```python
from build123d import *

# Parameters (mm, degrees)
SKETCH_1_R               = 40
EXTRUDE_1_DEPTH          = 5
SKETCH_2_R               = 31
EXTRUDE_2_DEPTH          = 12
SKETCH_3_R               = 26
CUT_EXTRUDE_1_DEPTH      = 15
SKETCH_4_R               = 31
EXTRUDE_3_DEPTH          = 3
SKETCH_6_R               = 2
CUT_EXTRUDE_3_DEPTH      = 5
PATTERN_CIRCULAR_1_COUNT = 4
SKETCH_7_R               = 20
CUT_EXTRUDE_4_DEPTH      = 10


with BuildPart() as part:
    # 草图1 → 凸台-拉伸1 (new body)
    with BuildSketch(Plane.XY):
        Circle(SKETCH_1_R)
    extrude(amount=EXTRUDE_1_DEPTH)

    # 草图2 → 凸台-拉伸2 (add)
    with BuildSketch(Plane.XY.offset(5)):
        Circle(SKETCH_2_R)
    extrude(amount=EXTRUDE_2_DEPTH)

    # 草图3 → 切除-拉伸1 (cut)
    with BuildSketch(Plane(origin=(0, 0, 0), x_dir=(-1, 0, 0), z_dir=(0, 0, -1))):
        Circle(SKETCH_3_R)
    extrude(amount=-CUT_EXTRUDE_1_DEPTH, mode=Mode.SUBTRACT)

    # 草图4 → 凸台-拉伸3 (add)
    with BuildSketch(Plane.XY.offset(17)):
        Circle(SKETCH_4_R)
    extrude(amount=EXTRUDE_3_DEPTH)

    # 草图6 → 切除-拉伸3 (cut)
    with BuildSketch(Plane(origin=(0, 0, 0), x_dir=(-1, 0, 0), z_dir=(0, 0, -1))):
        with Locations((0, 36)):
            Circle(SKETCH_6_R)
    cut_extrude_3 = extrude(amount=-CUT_EXTRUDE_3_DEPTH, mode=Mode.SUBTRACT)

    # 阵列(圆周)1: 切除-拉伸3 ×4 about axis
    pattern_circular_1_axis = Axis((0, 0, 0), (0, 0, 1))
    for i in range(1, PATTERN_CIRCULAR_1_COUNT):
        add(cut_extrude_3.rotate(pattern_circular_1_axis, i * 360 / PATTERN_CIRCULAR_1_COUNT), mode=Mode.SUBTRACT)

    # 草图7 → 切除-拉伸4 (cut)
    with BuildSketch(Plane.XY.offset(20)):
        Circle(SKETCH_7_R)
    extrude(amount=-CUT_EXTRUDE_4_DEPTH, mode=Mode.SUBTRACT)


solid = part.part
```
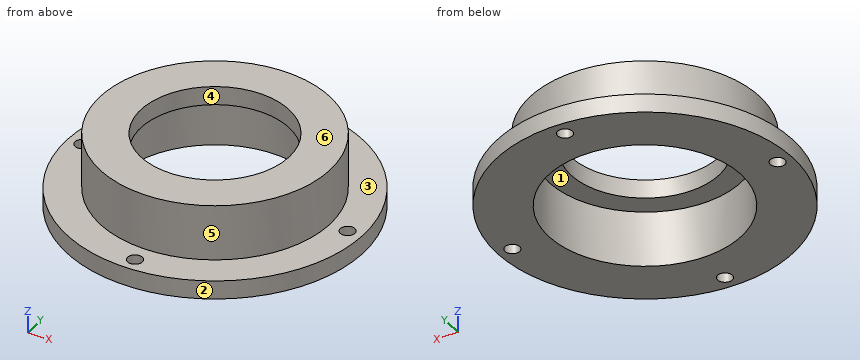
Geometry check sheet. Reference: the model listing, model coordinates, mm. Face numbers are marked on the shaded views. A direction names the side the tool comes from. Round coordinates to 2 decimals unless told otherwise and drop trailing zeros. Loops run counter-clockwise (first coordinate to the right, second up) from the corner with the lowest first, then second, coordinate; pieces in that order, holes last. Notation, with made-up numbers: (-21, 0.25) -> (25, 0.25) arc R16 ccw to (25, 22.25) -> close; hole circle Ø7 at (31, -16.5). An arc over 180 degrees is marked (long way). Use a Markdown table: item, result.
(1) Sectioned sample at C-C (z = 2.25). Enter the section's corners in (x, y), then the cut area to 3 significant figures.
Calculated:
| item | result |
|---|---|
| outline | circle Ø80 at (0, 0); hole circle Ø4 at (-36, 0); hole circle Ø52 at (0, 0); hole circle Ø4 at (0, -36); hole circle Ø4 at (0, 36); hole circle Ø4 at (36, 0) |
| area | 2,850 mm² |
(2) Scan lines: probe 1 along Y at (x, z) = (0, 4.5); probe 2 along Y at (x, z) = (0, 10); probe 3 along Z at (x, y) = (-24.5, 25). Record each from-to range of solid material in increasing order.
Calculated:
| item | result |
|---|---|
| probe 1 | -40 to -38, -34 to -26, 26 to 34, 38 to 40 |
| probe 2 | -31 to -26, 26 to 31 |
| probe 3 | 0 to 5 |
(3) Go/stop test with flat-tipped pins: P1, Ø5, axis at x = 26, z = 3.5, coming from the +Y side; P2, Ø8, axis at y = -4, z = 5, coming from the -X side; P3, Ø6.5, axis at x = 36, y = 0, coming from the +Z side; P4, Ø4, axis at x = 14, z = 8.5, coming from the +Y side. Record where each tip stops, or that it passes through.
Calculated:
| item | result |
|---|---|
| P1 | y = 32.37 |
| P2 | x = -40 |
| P3 | z = 5 |
| P4 | y = 28.58 |
(4) Sectioned sample at A-A (y = 0). Enter the section's corners in (x, z).
Calculated:
| item | result |
|---|---|
| outline | (-40, 0) -> (-38, 0) -> (-38, 5) -> (-40, 5) -> close; (-34, 0) -> (-26, 0) -> (-26, 15) -> (-20, 15) -> (-20, 20) -> (-31, 20) -> (-31, 5) -> (-34, 5) -> close; (20, 15) -> (26, 15) -> (26, 0) -> (34, 0) -> (34, 5) -> (31, 5) -> (31, 20) -> (20, 20) -> close; (38, 0) -> (40, 0) -> (40, 5) -> (38, 5) -> close |
(5) Sectioned sample at D-D (x = -15). Enter the section's corners in (y, z), then the cut area to 3 significant figures.
Calculated:
| item | result |
|---|---|
| outline | (-37.08, 0) -> (-21.24, 0) -> (-21.24, 15) -> (-13.23, 15) -> (-13.23, 20) -> (-27.13, 20) -> (-27.13, 5) -> (-37.08, 5) -> close; (13.23, 15) -> (21.24, 15) -> (21.24, 0) -> (37.08, 0) -> (37.08, 5) -> (27.13, 5) -> (27.13, 20) -> (13.23, 20) -> close |
| area | 415 mm² |
(6) Set-up check for the marked faces 1, 2 and 3: record each of +Z, -Z, +X, -X, +Y, -Y from which the full face is reachable in a straight line by a thin tool's end or side.
Calculated:
| item | result |
|---|---|
| face 1 | -Z |
| face 2 | +Z, -Z |
| face 3 | +Z |
(7) Mould release check, pull along Y, two halves, no side actions. Record for the marked faces 4, 5 and 6: released by +Y, released by -Y, zero draft, split by the parting line, or undercut.
Calculated:
| item | result |
|---|---|
| face 4 | undercut |
| face 5 | split by the parting line |
| face 6 | zero draft |
